The listing builds one solid part. Answer for the finished solid, in the listing's coordinates (mm). A direction names the side the tool comes from. Give positions to 0.01 mm unless a question says otherwise; leave off trailing zeros. Order: outer loops, then holes, each group sorted by start corner. A loop starts at its lowest first (then second) coordinate and runs counter-clockwise, first axis right, second up. Notation, with made-up numbers: (-15.5, -32) - (19.5, -32) arc R24 cw to (19.5, -10) - close; hole circle Ø8 at (83.5, 18.5). An arc over 180 degrees is marked (long way). Answer in a Markdown table with one row per item.
from build123d import *

# Parameters (mm, degrees)
F0_R     = 6
F0_W     = 40
F0_H     = 5
F1_DEPTH = 10


with BuildPart() as f1:
    # F0 (on Front) → F1 (new body)
    with BuildSketch(Plane.XZ):
        Polygon((0, 80), (0, 0), (80, 0), (80, 80), (60, 80), (20, 80), align=None)
        with Locations((26, 17)):
            Circle(F0_R, mode=Mode.SUBTRACT)
        with Locations((54, 17)):
            Circle(F0_R, mode=Mode.SUBTRACT)
        with Locations((26, 49)):
            Circle(F0_R, mode=Mode.SUBTRACT)
        with Locations((54, 49)):
            Circle(F0_R, mode=Mode.SUBTRACT)
        with Locations((40, 82.5)):
            Rectangle(F0_W, F0_H)
    extrude(amount=F1_DEPTH)


solid = f1.part
Item 1: Consider line 1 (Z direction, x = 53.5, y = -2); line 2 (X direction, y = -5.5, z = 14); line 3 (Z direction, x = 22.5, y = -2.5). Determine where each line is inside the solid, lowest interval first.
Answer block:
| item | result |
|---|---|
| line 1 | 0 to 11.02, 22.98 to 43.02, 54.98 to 85 |
| line 2 | 0 to 20.8, 31.2 to 48.8, 59.2 to 80 |
| line 3 | 0 to 12.13, 21.87 to 44.13, 53.87 to 85 |
Item 2: Find section A-A on z = 17. Write down the section's boundary in (x, y), then the cut area to 3 significant figures.
Answer block:
| item | result |
|---|---|
| outline | (0, -10) - (20, -10) - (20, 0) - (0, 0) - close; (32, -10) - (48, -10) - (48, 0) - (32, 0) - close; (60, -10) - (80, -10) - (80, 0) - (60, 0) - close |
| area | 560 mm² |
Item 3: This flat-tipped pin is pushed along its axis until it touches: P1, Ø14, axis at x = 54, z = 49, coming from the -Y side. Where does it stop, or does it pass through?
Answer block:
| item | result |
|---|---|
| P1 | y = -10 |
Item 4: Find section C-C on y = -8. Write down the section's boundary in (x, z), then the cut area to 3 significant figures.
Answer block:
| item | result |
|---|---|
| outline | (0, 0) - (80, 0) - (80, 80) - (60, 80) - (60, 85) - (20, 85) - (20, 80) - (0, 80) - close; hole circle Ø12 at (26, 17); hole circle Ø12 at (26, 49); hole circle Ø12 at (54, 17); hole circle Ø12 at (54, 49) |
| area | 6,150 mm² |
Item 5: Determine the mould class of faces 4 (the face through (48, -5, 49)), 5 (the face through (20, -5, 82)), 6 (the face through (70, -5, 80)) for opening direction Z: pulls with the +Z half, pulls with the -Z half, needs draft (parallel to the pull), parting line crosses it, or undercut.
Answer block:
| item | result |
|---|---|
| face 4 | undercut |
| face 5 | needs draft |
| face 6 | pulls with the +Z half |
Item 6: Find section B-B on x = 26. Write down the section's boundary in (y, z).
Answer block:
| item | result |
|---|---|
| outline | (-10, 0) - (0, 0) - (0, 11) - (-10, 11) - close; (-10, 23) - (0, 23) - (0, 43) - (-10, 43) - close; (-10, 55) - (0, 55) - (0, 85) - (-10, 85) - close |
Item 7: Find section D-D on x = 10.5. Write down the section's boundary in (y, z), then the cut area to 3 significant figures.
Answer block:
| item | result |
|---|---|
| outline | (-10, 0) - (0, 0) - (0, 80) - (-10, 80) - close |
| area | 800 mm² |
Item 8: Which of the six approach directions +Z, -Z, +X, -X, +Y, -Y give full straight-line access (tool end or side, diameter ignored) to faces 1 (the face through (39, 0, 43)), 2 (the face through (60, -5, 82)), 3 (the face through (10, -5, 80))?
Answer block:
| item | result |
|---|---|
| face 1 | +Z, -Z, +X, -X, +Y |
| face 2 | +Z, +X, +Y, -Y |
| face 3 | +Z, -X, +Y, -Y |
